from build123d import *

# Parameters (mm, degrees)
SKETCH1_W                               = 304.8
SKETCH1_H                               = 86.36
BOSS_EXTRUDE1_DEPTH                     = 3.175
F_1_8_0_125_PRESS_DOWEL_HOLE1_OUTLINE_R = 1.5875
F_1_8_0_125_PRESS_DOWEL_HOLE1_DEPTH     = 3.175
CUT_EXTRUDE1_DEPTH                      = 317.814094107
SKETCH7_W                               = 19.05
SKETCH7_H                               = 25.4
SKETCH7_H_2                             = 71.12
CUT_EXTRUDE2_DEPTH                      = 317.814094107
FILLET1_R                               = 3.175
F_1_2_0_5_PRESS_DOWEL_HOLE1_D           = 12.7
F_3_0MM_PRESS_DOWEL_HOLE1_D             = 3
F_3_0MM_PRESS_DOWEL_HOLE1_DEPTH         = 3.175
F_3_0MM_PRESS_DOWEL_HOLE1_TIP           = 0.901290929
F_2_0MM_PRESS_DOWEL_HOLE1_D             = 2
F_2_0MM_PRESS_DOWEL_HOLE1_DEPTH         = 3.175
F_2_0MM_PRESS_DOWEL_HOLE1_TIP           = 0.600860619
F_4_40_TAPPED_HOLE2_D                   = 2.2606
F_1_8_0_125_DIAMETER_HOLE1_D            = 3.175


# Read off the part's stored shape, not the designer's step: 1/8 (0.125) Press Dowel Hole1
with BuildPart() as part:
    # Sketch1 → Boss-Extrude1 (new body)
    with BuildSketch(Plane(origin=(0, 0, 0), x_dir=(0, 0, -1), z_dir=(1, 0, 0))):
        with Locations((152.4, 43.18)):
            Rectangle(SKETCH1_W, SKETCH1_H)
    extrude(amount=BOSS_EXTRUDE1_DEPTH)

    # 1/8 (0.125) Press Dowel Hole1 outline → 1/8 (0.125) Press Dowel Hole1 (cut)
    with BuildSketch(Plane.YZ):
        with Locations((68.36, -269.24)):
            Circle(F_1_8_0_125_PRESS_DOWEL_HOLE1_OUTLINE_R)
        with Locations((18, -269.24)):
            Circle(F_1_8_0_125_PRESS_DOWEL_HOLE1_OUTLINE_R)
        with Locations((82.55, -25.4)):
            Circle(F_1_8_0_125_PRESS_DOWEL_HOLE1_OUTLINE_R)
        with Locations((82.55, -88.9)):
            Circle(F_1_8_0_125_PRESS_DOWEL_HOLE1_OUTLINE_R)
        with Locations((82.55, -190.5)):
            Circle(F_1_8_0_125_PRESS_DOWEL_HOLE1_OUTLINE_R)
        with Locations((82.55, -254)):
            Circle(F_1_8_0_125_PRESS_DOWEL_HOLE1_OUTLINE_R)
        with Locations((3.81, -254)):
            Circle(F_1_8_0_125_PRESS_DOWEL_HOLE1_OUTLINE_R)
        with Locations((3.81, -190.5)):
            Circle(F_1_8_0_125_PRESS_DOWEL_HOLE1_OUTLINE_R)
        with Locations((3.81, -88.9)):
            Circle(F_1_8_0_125_PRESS_DOWEL_HOLE1_OUTLINE_R)
        with Locations((3.81, -25.4)):
            Circle(F_1_8_0_125_PRESS_DOWEL_HOLE1_OUTLINE_R)
    extrude(amount=F_1_8_0_125_PRESS_DOWEL_HOLE1_DEPTH, mode=Mode.SUBTRACT)

    # Sketch6 → Cut-Extrude1 (cut, through all)
    with BuildSketch(Plane(origin=(3.175, 0, 0), x_dir=(0, 0, -1), z_dir=(1, 0, 0))):
        with BuildLine():
            Line((141.5288, 73.66), (141.5288, 56.781492032))
            ThreePointArc((141.5288, 56.781492032), (139.7, 54.952692032), (137.8712, 56.781492032))
            Line((137.8712, 56.781492032), (137.8712, 73.66))
            ThreePointArc((137.8712, 73.66), (139.7, 75.4888), (141.5288, 73.66))
        make_face()
        with BuildLine():
            Line((141.5288, 12.7), (141.5288, 29.578507968))
            ThreePointArc((141.5288, 29.578507968), (139.7, 31.407307968), (137.8712, 29.578507968))
            Line((137.8712, 29.578507968), (137.8712, 12.7))
            ThreePointArc((137.8712, 12.7), (139.7, 10.8712), (141.5288, 12.7))
        make_face()
    extrude(amount=-CUT_EXTRUDE1_DEPTH, mode=Mode.SUBTRACT)

    # Sketch7 → Cut-Extrude2 (cut, through all)
    with BuildSketch(Plane(origin=(3.175, 0, 0), x_dir=(0, 0, -1), z_dir=(1, 0, 0))):
        Polygon((7.62, 73.66), (7.62, 12.7), (50.8, 43.18), align=None)
        with Locations((287.655, 66.04)):
            Rectangle(SKETCH7_W, SKETCH7_H)
        Polygon((100.33, 12.7), (57.15, 43.18), (100.33, 73.66), align=None)
        with Locations((161.925, 43.18)):
            Rectangle(SKETCH7_W, SKETCH7_H_2)
        Polygon((179.07, 25.4), (224.15112849, 43.18), (179.07, 60.96), align=None)
        Polygon((53.975, 73.66), (88.265, 73.66), (53.975, 49.455294118), (19.685, 73.66), align=None)
        Polygon((53.975, 36.904705882), (19.685, 12.7), (53.975, 12.7), (88.265, 12.7), align=None)
        Polygon((179.07, 12.7), (217.710967277, 27.94), (237.51919806, 27.94), (266.065, 19.05), (266.065, 12.7), (225.425, 12.7), align=None)
        Polygon((217.710967277, 58.42), (237.51919806, 58.42), (266.065, 67.31), (266.065, 73.66), (225.425, 73.66), (179.07, 73.66), align=None)
        with Locations((287.655, 20.32)):
            Rectangle(SKETCH7_W, SKETCH7_H)
        with Locations((117.475, 43.18)):
            Rectangle(SKETCH7_W, SKETCH7_H_2)
    extrude(amount=-CUT_EXTRUDE2_DEPTH, mode=Mode.SUBTRACT)

    # Fillet1
    fillet1_edges = [part.edges().sort_by_distance(p)[0] for p in [
        (1.5875, 73.66, -7.62),
        (1.5875, 43.18, -50.8),
        (1.5875, 12.7, -7.62),
        (1.5875, 53.34, -278.13),
        (1.5875, 78.74, -278.13),
        (1.5875, 78.74, -297.18),
        (1.5875, 53.34, -297.18),
        (1.5875, 73.66, -100.33),
        (1.5875, 12.7, -100.33),
        (1.5875, 43.18, -57.15),
        (1.5875, 12.7, -179.07),
        (1.5875, 27.94, -217.710967277),
        (1.5875, 27.94, -237.51919806),
        (1.5875, 19.05, -266.065),
        (1.5875, 12.7, -266.065),
        (1.5875, 25.4, -179.07),
        (1.5875, 60.96, -179.07),
        (1.5875, 43.18, -224.15112849),
        (1.5875, 73.66, -19.685),
        (1.5875, 73.66, -88.265),
        (1.5875, 49.455294118, -53.975),
        (1.5875, 36.904705882, -53.975),
        (1.5875, 12.7, -88.265),
        (1.5875, 12.7, -19.685),
        (1.5875, 73.66, -266.065),
        (1.5875, 67.31, -266.065),
        (1.5875, 58.42, -237.51919806),
        (1.5875, 58.42, -217.710967277),
        (1.5875, 73.66, -179.07),
        (1.5875, 7.62, -152.4),
        (1.5875, 78.74, -152.4),
        (1.5875, 78.74, -171.45),
        (1.5875, 7.62, -171.45),
        (1.5875, 7.62, -278.13),
        (1.5875, 33.02, -278.13),
        (1.5875, 33.02, -297.18),
        (1.5875, 7.62, -297.18),
        (1.5875, 7.62, -107.95),
        (1.5875, 78.74, -107.95),
        (1.5875, 78.74, -127),
        (1.5875, 7.62, -127),
    ]]
    fillet(fillet1_edges, radius=FILLET1_R)

    # 1/2 (0.5) Press Dowel Hole1 (through all)
    with Locations(Plane.ZY):
        with Locations((-248.01972494, 46.53348834)):
            Hole(F_1_2_0_5_PRESS_DOWEL_HOLE1_D / 2)

    # Ø3.0mm Press Dowel Hole1
    with Locations(Plane.ZY):
        with Locations((-253.55249518, 29.46260554)):
            Hole(F_3_0MM_PRESS_DOWEL_HOLE1_D / 2, depth=F_3_0MM_PRESS_DOWEL_HOLE1_DEPTH)
            with Locations((0, 0, -(F_3_0MM_PRESS_DOWEL_HOLE1_DEPTH + F_3_0MM_PRESS_DOWEL_HOLE1_TIP / 2))):  # 118° drill point
                Cone(0, F_3_0MM_PRESS_DOWEL_HOLE1_D / 2, F_3_0MM_PRESS_DOWEL_HOLE1_TIP, mode=Mode.SUBTRACT)

    # Ø2.0mm Press Dowel Hole1
    with Locations(Plane.ZY):
        with Locations((-267.20941224, 24.95127344)):
            Hole(F_2_0MM_PRESS_DOWEL_HOLE1_D / 2, depth=F_2_0MM_PRESS_DOWEL_HOLE1_DEPTH)
            with Locations((0, 0, -(F_2_0MM_PRESS_DOWEL_HOLE1_DEPTH + F_2_0MM_PRESS_DOWEL_HOLE1_TIP / 2))):  # 118° drill point
                Cone(0, F_2_0MM_PRESS_DOWEL_HOLE1_D / 2, F_2_0MM_PRESS_DOWEL_HOLE1_TIP, mode=Mode.SUBTRACT)

    # #4-40 Tapped Hole2 (through all)
    with Locations(Plane(origin=(3.175, 0, 0), x_dir=(0, 0, -1), z_dir=(1, 0, 0))):
        with Locations((301.625, 81.2038), (301.625, 5.1562), (3.175, 81.2038), (3.175, 5.1562), (175.26, 66.04), (175.26, 20.32), (104.14, 66.04), (104.14, 20.32)):
            Hole(F_4_40_TAPPED_HOLE2_D / 2)

    # 1/8 (0.125) Diameter Hole1 (through all)
    with Locations(Plane(origin=(3.175, 0, 0), x_dir=(0, 0, -1), z_dir=(1, 0, 0))):
        with Locations((278.835955069, 43.18)):
            Hole(F_1_8_0_125_DIAMETER_HOLE1_D / 2)


solid = part.part
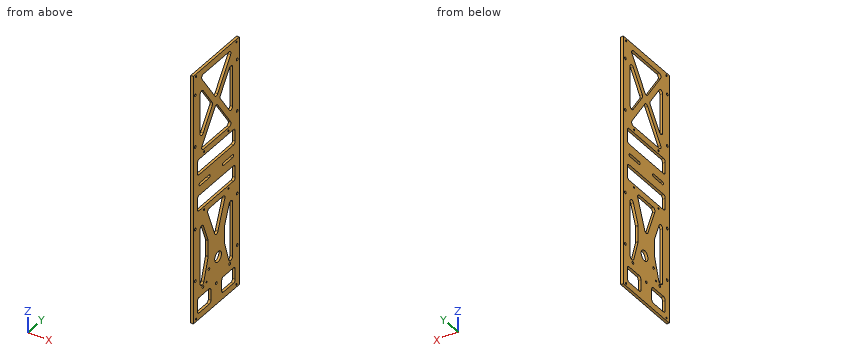
Read the model definition and answer for the solid it produces. Units are mm, in the model's axes. Give positions to 0.01 mm unless a question says otherwise; leave off trailing zeros. Answer as a JSON object with one key per item and string values. Group by question number.
1) This flat-tipped pin is pushed along its axis until it touches: P1, Ø5, axis at y = 29.46, z = -253.55, coming from the -X side. Where does it stop, or does it pass through?
2) Find section A-A (x = 1.3). Count the separate pieces of the cut face and the enclosed holes in it, and give its area (3 significant figures).
3) Consider L1, parallel to Y at x = 3.05, z = -258.5; L2, parallel to Y at x = 1.35, z = -190.5; L3, parallel to Y at x = 3, z = -166.5. Determine where each line is inside the solid, lowest interval first. Write a range as from..to.
Values follow:
{
 "1": {"P1": "stops at x = 0"},
 "2": {"separate pieces": "1", "enclosed holes": "35", "area": "15,600 mm2"},
 "3": {"L1": "y = 0..12.7, 21.41..64.95, 73.66..86.36", "L2": "y = 0..2.22, 5.4..29.91, 56.45..80.96, 84.14..86.36", "L3": "y = 0..7.62, 78.74..86.36"}
}
